For this review, take the finished solid that the model builds, in its own axes (mm). Face numbers are marked on the shaded views. Round coordinates to 2 decimals unless told otherwise and drop trailing zeros. Order: outer loops, then holes, each group sorted by start corner. A loop starts at its lowest first (then second) coordinate and runs counter-clockwise, first axis right, second up. Notation, with made-up numbers: (-39.75, 69.25) - (2.25, 69.25) arc R18 ccw to (2.25, 86.25) - close; hole circle Ø7 at (24.5, 14.5). An arc over 180 degrees is marked (long way). One line per item, written item: value.
```python
from build123d import *

# Parameters (mm, degrees)
CROQUIS1_W                         = 20
CROQUIS1_H                         = 50.8
BRIDA_BASE1_DEPTH                  = 1
BRIDA_DE_ARISTA1_STRIP_W           = 5.4732
BRIDA_DE_ARISTA1_STRIP_H           = 1
BRIDA_DE_ARISTA1_STRIP_CUT_DEPTH   = 50.8
BRIDA_DE_ARISTA1_STRIP_2_W         = 5.4732
BRIDA_DE_ARISTA1_STRIP_2_H         = 1
BRIDA_DE_ARISTA1_STRIP_CUT_2_DEPTH = 50.8
BRIDA_DE_ARISTA1_DEPTH             = 50.8
BRIDA_DE_ARISTA1_BEND_DEPTH        = 50.8
CROQUIS14_W                        = 15
CROQUIS14_H                        = 50
PESTA_A1_DEPTH                     = 1
CROQUIS17_R                        = 3
CORTAR_EXTRUIR1_DEPTH              = 89.14283862
REDONDEO1_R                        = 10
REDONDEO2_R                        = 7.5


# Sheet-metal steps are written as plain solids
with BuildPart() as part:
    # Croquis1 → Brida base1 (new body)
    with BuildSketch(Plane.XY):
        Rectangle(CROQUIS1_W, CROQUIS1_H)
    extrude(amount=-BRIDA_BASE1_DEPTH)

    # Brida de arista1 strip (across the edge) → Brida de arista1 strip cut (cut)
    with BuildSketch(Plane(origin=(-10, 25.4, 0), x_dir=(1, 0, 0), z_dir=(0, -1, 0))):
        with Locations((-2, -0.5)):
            Rectangle(BRIDA_DE_ARISTA1_STRIP_W, BRIDA_DE_ARISTA1_STRIP_H)
    extrude(amount=BRIDA_DE_ARISTA1_STRIP_CUT_DEPTH, mode=Mode.SUBTRACT)

    # Brida de arista1 strip 2 (across the edge) → Brida de arista1 strip cut 2 (cut)
    with BuildSketch(Plane(origin=(10, -25.4, 0), x_dir=(-1, 0, 0), z_dir=(0, 1, 0))):
        with Locations((-2, -0.5)):
            Rectangle(BRIDA_DE_ARISTA1_STRIP_2_W, BRIDA_DE_ARISTA1_STRIP_2_H)
    extrude(amount=BRIDA_DE_ARISTA1_STRIP_CUT_2_DEPTH, mode=Mode.SUBTRACT)

    # Brida de arista1 section (across the edge) → Brida de arista1 (add)
    with BuildSketch(Plane(origin=(-10, 25.4, 0), x_dir=(1, 0, 0), z_dir=(0, -1, 0))):
        with BuildLine():
            Line((-1, 0.7366), (-1, 40))
            Line((-1, 40), (0, 40))
            Line((0, 40), (0, 0.7366))
            ThreePointArc((0, 0.7366), (0.215745145, 0.215745145), (0.7366, 0))
            Line((0.7366, 0), (0.7366, -1))
            ThreePointArc((0.7366, -1), (-0.491361636, -0.491361636), (-1, 0.7366))
        make_face()
    extrude(amount=BRIDA_DE_ARISTA1_DEPTH)

    # Brida de arista1 section 2 (across the edge) → Brida de arista1 bend (add)
    with BuildSketch(Plane(origin=(10, -25.4, 0), x_dir=(-1, 0, 0), z_dir=(0, 1, 0))):
        with BuildLine():
            Line((-1, 0.7366), (-1, 40))
            Line((-1, 40), (0, 40))
            Line((0, 40), (0, 0.7366))
            ThreePointArc((0, 0.7366), (0.215745145, 0.215745145), (0.7366, 0))
            Line((0.7366, 0), (0.7366, -1))
            ThreePointArc((0.7366, -1), (-0.491361636, -0.491361636), (-1, 0.7366))
        make_face()
    extrude(amount=BRIDA_DE_ARISTA1_BEND_DEPTH)

    # Croquis14 → Pestaña1 (add)
    with BuildSketch(Plane.ZY.offset(11)):
        with Locations((32.5, -50.4)):
            Rectangle(CROQUIS14_W, CROQUIS14_H)
    pesta_a1 = extrude(amount=-PESTA_A1_DEPTH)

    # Simetría1: Pestaña1 across plane
    add(pesta_a1.mirror(Plane(origin=(0, 0, 0), x_dir=(0, 0, 1), z_dir=(1, 0, 0))))

    # Croquis17 → Cortar-Extruir1 (cut, through all)
    with BuildSketch(Plane.ZY.offset(11)):
        with Locations((33.4285, -67.4)):
            Circle(CROQUIS17_R)
    extrude(amount=-CORTAR_EXTRUIR1_DEPTH, mode=Mode.SUBTRACT)

    # Redondeo1
    redondeo1_edges = [part.edges().sort_by_distance(p)[0] for p in [
        (-10.5, 25.4, 40),
        (10.5, 25.4, 40),
        (-10.5, -25.4, 25),
        (10.5, -25.4, 25),
    ]]
    fillet(redondeo1_edges, radius=REDONDEO1_R)

    # Redondeo2
    redondeo2_edges = [part.edges().sort_by_distance(p)[0] for p in [
        (10.5, -75.4, 25),
        (10.5, -75.4, 40),
        (-10.5, -75.4, 25),
        (-10.5, -75.4, 40),
    ]]
    fillet(redondeo2_edges, radius=REDONDEO2_R - 0.0001)  # a hair under: the kernel refuses the full size


solid = part.part
```
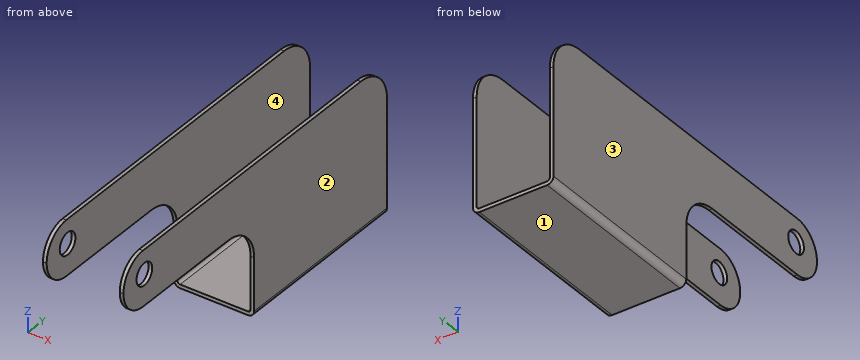
Item 1: Take a section at A-A (y = -58.5). Write out the cut boundary in (x, z), plus the area to 3 significant figures.
Returned:
outline: (-11, 25) - (-10, 25) - (-10, 40) - (-11, 40) - close; (10, 25) - (11, 25) - (11, 40) - (10, 40) - close
area: 30.0 mm^2
Item 2: Take a section at B-B (z = 4). Write out the cut boundary in (x, y).
Returned:
outline: (-11, -25.4) - (-10, -25.4) - (-10, 25.4) - (-11, 25.4) - close; (10, -25.4) - (11, -25.4) - (11, 25.4) - (10, 25.4) - close
Item 3: Take a section at D-D (x = 7.5). Write out the cut boundary in (y, z).
Returned:
outline: (-25.4, -1) - (25.4, -1) - (25.4, 0) - (-25.4, 0) - close
Item 4: Wall thickness on line 1 (X direction, y = -7.5, z = 15); line 2 (Z direction, x = -8, y = 9.5): over which ranges is each line inside the solid? List them lowest first.
Returned:
line 1: -11 to -10, 10 to 11
line 2: -1 to 0
Item 5: For P1, Ø13, axis at x = -2, z = 3, coming from the -Y side; P2, Ø1.1, axis at x = -10.5, y = -56, coming from the -Z side, all flat-tipped, find the tip position at first contact; note any pin that passes through.
Returned:
P1: y = -25.4
P2: z = 25
Item 6: Take a section at C-C (y = -2). Write out the cut boundary in (x, z), plus the area to 3 significant figures.
Returned:
outline: (-11, 0.74) arc R1.74 ccw to (-9.26, -1) - (9.26, -1) arc R1.74 ccw to (11, 0.74) - (11, 40) - (10, 40) - (10, 0.74) arc R0.74 cw to (9.26, 0) - (-9.26, 0) arc R0.74 cw to (-10, 0.74) - (-10, 40) - (-11, 40) - close
area: 101 mm^2
Item 7: The part is to be moulded in two halves that separate along X. For the marked faces 1, 2, 3 and 4, say which applies: +X half, -X half, draft (parallel to the pull), parting line (faces both ways), or undercut.
Returned:
face 1: draft
face 2: +X half
face 3: -X half
face 4: undercut
